The listing builds one solid part. Answer for the finished solid, in the listing's coordinates (mm). A direction names the side the tool comes from. Give positions to 0.01 mm unless a question says otherwise; leave off trailing zeros. Order: outer loops, then holes, each group sorted by start corner. A loop starts at its lowest first (then second) coordinate and runs counter-clockwise, first axis right, second up. Notation, with made-up numbers: (57.25, 61.5) - (68.25, 61.5) arc R30 ccw to (68.25, 92.5) - close; hole circle Ø7 at (21.25, -27). An arc over 180 degrees is marked (long way). Answer as a JSON object with one key per item and string values. Group by question number.
Q1. Consider line 1 (Z direction, x = -13, y = -7.5); line 2 (Y direction, x = 0, z = 8.5); line 3 (Y direction, x = 0, z = -13). Determine where each line is inside the solid, lowest interval first.
Q2. The mould has two halves that part along Z. Classify faces 1 (the face through (7, 0, -16)), 2 (the face through (-0.07, -14.15, 3)), 3 (the face through (-3.47, -15.62, 10.58)), 4 (the face through (-0.07, -14.15, -5)): released by +Z, released by -Z, zero draft, split by the parting line, or undercut.
Q3. A cutting plane is placed at D-D, the plane y = -6. Give the vertices of the cut face in (x, z).
Q4. A cutting plane is placed at A-A, the plane x = 0. Give the vertices of the cut face in (y, z), and give its area (3 significant figures).
Q5. For faces 5 (the face through (-5.198, 1.637, -11.07)), 6 (the face through (-3.47, -15.62, -10.42)), 7 (the face through (12.932, -5.362, -3.986)), determine the directions among +Z, -Z, +X, -X, +Y, -Y from which every point of the face is accessible in a straight line to the end or side of a thin tool.
Q6. A cutting plane is placed at B-B, the plane y = 3. Give the vertices of the cut face in (x, z).
Q7. Given pin 1 (4 mm diameter, centred on y = 7.5, z = 4.5, fed in from +X); pin 2 (8.5 mm diameter, centred on x = -2.5, y = -2, fed in from -Z); pin 3 (12 mm diameter, centred on x = 7.5, z = 12, fed in from +Y); pin 4 (3 mm diameter, centred on x = -4.5, z = -1.5, fed in from +Y), each flat-ended and moving along its own axis, determine where each tip first touches the part or whether it passes through.
Q8. A cutting plane is placed at C-C, the plane z = 7.5. Give the vertices of the cut face in (x, y), and give its area (3 significant figures).
from build123d import *

# Parameters (mm, degrees)
SKETCH_1_R          = 16
SKETCH_1_R_2        = 4
EXTRUDE_1_DEPTH     = 16
CUT_EXTRUDE_START   = 5
SKETCH_2_R          = 16
SKETCH_2_R_2        = 14
CUT_EXTRUDE_1_DEPTH = 2
CUT_EXTRUDE_START_2 = -3
SKETCH_2_2_R        = 16
SKETCH_2_2_R_2      = 14
CUT_EXTRUDE_2_DEPTH = 2
SKETCH_4_R          = 5.45
CUT_EXTRUDE_4_DEPTH = 10


with BuildPart() as part:
    # 스케치1 → 보스-돌출1 (new, symmetric)
    with BuildSketch(Plane.XY):
        Circle(SKETCH_1_R)
        Circle(SKETCH_1_R_2, mode=Mode.SUBTRACT)
    extrude(amount=EXTRUDE_1_DEPTH, both=True)

    # 스케치2 → 컷-돌출1 (cut)
    with BuildSketch(Plane.XY.offset(CUT_EXTRUDE_START)):
        Circle(SKETCH_2_R)
        Circle(SKETCH_2_R_2, mode=Mode.SUBTRACT)
    extrude(amount=-CUT_EXTRUDE_1_DEPTH, mode=Mode.SUBTRACT)

    # 스케치2<2> → 컷-돌출2 (cut)
    with BuildSketch(Plane.XY.offset(CUT_EXTRUDE_START_2)):
        Circle(SKETCH_2_2_R)
        Circle(SKETCH_2_2_R_2, mode=Mode.SUBTRACT)
    extrude(amount=-CUT_EXTRUDE_2_DEPTH, mode=Mode.SUBTRACT)

    # 스케치4 → 컷-돌출4 (cut)
    with BuildSketch(Plane(origin=(0, 0, -16), x_dir=(-1, 0, 0), z_dir=(0, 0, -1))):
        Circle(SKETCH_4_R)
    extrude(amount=-CUT_EXTRUDE_4_DEPTH, mode=Mode.SUBTRACT)


solid = part.part
Reply:
{
 "1": {"line 1": "z = -16 to -5, -3 to 3, 5 to 16", "line 2": "y = -16 to -4, 4 to 16", "line 3": "y = -16 to -5.45, 5.45 to 16"},
 "2": {"face 1": "released by -Z", "face 2": "undercut", "face 3": "zero draft", "face 4": "undercut"},
 "3": {"outline": "(-14.83, -16) - (14.83, -16) - (14.83, -5) - (12.65, -5) - (12.65, -3) - (14.83, -3) - (14.83, 3) - (12.65, 3) - (12.65, 5) - (14.83, 5) - (14.83, 16) - (-14.83, 16) - (-14.83, 5) - (-12.65, 5) - (-12.65, 3) - (-14.83, 3) - (-14.83, -3) - (-12.65, -3) - (-12.65, -5) - (-14.83, -5) - close"},
 "4": {"outline": "(-16, -16) - (-5.45, -16) - (-5.45, -6) - (-4, -6) - (-4, 16) - (-16, 16) - (-16, 5) - (-14, 5) - (-14, 3) - (-16, 3) - (-16, -3) - (-14, -3) - (-14, -5) - (-16, -5) - close; (4, -6) - (5.45, -6) - (5.45, -16) - (16, -16) - (16, -5) - (14, -5) - (14, -3) - (16, -3) - (16, 3) - (14, 3) - (14, 5) - (16, 5) - (16, 16) - (4, 16) - close", "area": "723 mm^2"},
 "5": {"face 5": "-Z", "face 6": "+Z, -Z", "face 7": "none"},
 "6": {"outline": "(-15.72, -16) - (-4.55, -16) - (-4.55, -6) - (-2.65, -6) - (-2.65, 16) - (-15.72, 16) - (-15.72, 5) - (-13.67, 5) - (-13.67, 3) - (-15.72, 3) - (-15.72, -3) - (-13.67, -3) - (-13.67, -5) - (-15.72, -5) - close; (2.65, -6) - (4.55, -6) - (4.55, -16) - (15.72, -16) - (15.72, -5) - (13.67, -5) - (13.67, -3) - (15.72, -3) - (15.72, 3) - (13.67, 3) - (13.67, 5) - (15.72, 5) - (15.72, 16) - (2.65, 16) - close"},
 "7": {"pin 1": "stops at x = 15", "pin 2": "stops at z = -16", "pin 3": "stops at y = 15.93", "pin 4": "stops at y = 15.72"},
 "8": {"outline": "circle Ø32 at (0, 0); hole circle Ø8 at (0, 0)", "area": "754 mm^2"}
}
